```python
from build123d import *

# Parameters (mm, degrees)
BOSS_EXTRUDE1_DEPTH = 40
SKETCH2_R           = 2.1
CUT_EXTRUDE1_DEPTH  = 40
SKETCH3_R           = 2.1
CUT_EXTRUDE2_DEPTH  = 40
BOSS_EXTRUDE2_DEPTH = 4
BOSS_EXTRUDE3_DEPTH = 4


with BuildPart() as part:
    # Sketch1 → Boss-Extrude1 (new body)
    with BuildSketch(Plane(origin=(0, 0, 0), x_dir=(1, 0, 0), z_dir=(0, 1, 0))):
        Polygon((0, 0), (0, 40), (-40, 40), (-40, 36), (-4, 36), (-4, 0), align=None)
    extrude(amount=BOSS_EXTRUDE1_DEPTH)

    # Sketch2 → Cut-Extrude1 (cut)
    with BuildSketch(Plane(origin=(0, 0, -40), x_dir=(-1, 0, 0), z_dir=(0, 0, -1))):
        with Locations((30, 30)):
            Circle(SKETCH2_R)
        with Locations((30, 10)):
            Circle(SKETCH2_R)
        with Locations((10, 10)):
            Circle(SKETCH2_R)
        with Locations((10, 30)):
            Circle(SKETCH2_R)
    extrude(amount=-CUT_EXTRUDE1_DEPTH, mode=Mode.SUBTRACT)

    # Sketch3 → Cut-Extrude2 (cut)
    with BuildSketch(Plane(origin=(0, 0, 0), x_dir=(0, 0, -1), z_dir=(1, 0, 0))):
        with Locations((10, 30)):
            Circle(SKETCH3_R)
        with Locations((30, 30)):
            Circle(SKETCH3_R)
        with Locations((30, 10)):
            Circle(SKETCH3_R)
        with Locations((10, 10)):
            Circle(SKETCH3_R)
    extrude(amount=-CUT_EXTRUDE2_DEPTH, mode=Mode.SUBTRACT)

    # Sketch4 → Boss-Extrude2 (add)
    with BuildSketch(Plane(origin=(0, 40, 0), x_dir=(1, 0, 0), z_dir=(0, 1, 0))):
        Polygon((-40, 36), (-4, 0), (-4, 36), align=None)
    extrude(amount=-BOSS_EXTRUDE2_DEPTH)

    # Sketch5 → Boss-Extrude3 (add)
    with BuildSketch(Plane.XZ):
        Polygon((-4, -36), (-4, 0), (-40, -36), align=None)
    extrude(amount=-BOSS_EXTRUDE3_DEPTH)


solid = part.part
```
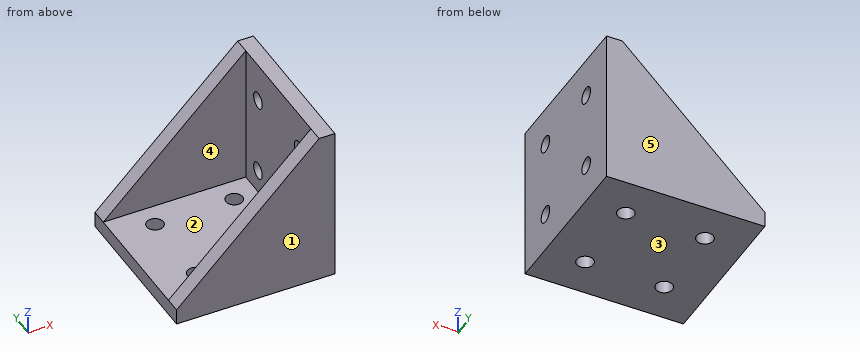
Check sheet for the modelled part. Datum: model origin and axes. Units: mm. Face numbers are marked on the shaded views. A direction names the side the tool comes from. Round coordinates to 2 decimals unless told otherwise and drop trailing zeros. Loops run counter-clockwise (first coordinate to the right, second up) from the corner with the lowest first, then second, coordinate; pieces in that order, holes last. Notation, with made-up numbers: (7.5, 14.5) -> (36.5, 14.5) arc R26 cw to (36.5, 46.5) -> close; hole circle Ø4 at (-19.5, 2.25). An arc over 180 degrees is marked (long way). Write item = value, one per line. Start each with the question number.
1) Release check for a two-part mould opening along Y. For the marked faces 3, 4 and 5 record: released by +Y, released by -Y, zero draft, split by the parting line, or undercut.
2) Thickness scan on probe 1 along Y at (x, z) = (-2.7, -30); probe 2 along Y at (x, z) = (-12, -22.5); probe 3 along X at (y, z) = (16.5, -10). Record the ranges inside material, lowest first.
3) Sectioned sample at C-C, the plane x = -30. Record the cut outline in (y, z), plus the area to 3 significant figures.
4) Set-up check for the marked faces 1 and 2: record each of +Z, -Z, +X, -X, +Y, -Y from which the full face is reachable in a straight line by a thin tool's end or side.
5) Sectioned sample at D-D, the plane x = -25. Record the cut outline in (y, z), plus the area to 3 significant figures.
6) Sectioned sample at A-A, the plane y = 10. Record the cut outline in (x, z).
7) Sectioned sample at B-B, the plane z = -10. Record the cut outline in (x, y).
8) Gauge pin test, flat ends, axial feed: pin 1 Ø10 at (x, y) = (-30, 28.5) entering from +Z; pin 2 Ø4 at (y, z) = (11, -19.5) entering from -X. Record the tip position at first contact, or that the pin passes through.
Results are:
q1.face_3 = zero draft
q1.face_4 = undercut
q1.face_5 = released by +Y
q2.probe_1 = 0 to 7.9, 12.1 to 27.9, 32.1 to 40
q2.probe_2 = 0 to 4, 36 to 40
q2.probe_3 = -4 to 0
q3.outline = (0, -40) -> (7.9, -40) -> (7.9, -36) -> (4, -36) -> (4, -26) -> (0, -26) -> close; (12.1, -40) -> (27.9, -40) -> (27.9, -36) -> (12.1, -36) -> close; (32.1, -40) -> (40, -40) -> (40, -26) -> (36, -26) -> (36, -36) -> (32.1, -36) -> close
q3.area = 206 mm^2
q4.face_1 = +Z, -Z, +X, -X, -Y
q4.face_2 = +Z, -X
q5.outline = (0, -40) -> (40, -40) -> (40, -21) -> (36, -21) -> (36, -36) -> (4, -36) -> (4, -21) -> (0, -21) -> close
q5.area = 280 mm^2
q6.outline = (-40, -40) -> (-32.1, -40) -> (-32.1, -36) -> (-40, -36) -> close; (-27.9, -40) -> (-12.1, -40) -> (-12.1, -36) -> (-27.9, -36) -> close; (-7.9, -40) -> (0, -40) -> (0, -32.1) -> (-4, -32.1) -> (-4, -36) -> (-7.9, -36) -> close; (-4, -27.9) -> (0, -27.9) -> (0, -12.1) -> (-4, -12.1) -> close; (-4, -7.9) -> (0, -7.9) -> (0, 0) -> (-4, 0) -> close
q7.outline = (-14, 0) -> (0, 0) -> (0, 7.9) -> (-4, 7.9) -> (-4, 4) -> (-14, 4) -> close; (-14, 36) -> (-4, 36) -> (-4, 32.1) -> (0, 32.1) -> (0, 40) -> (-14, 40) -> close; (-4, 12.1) -> (0, 12.1) -> (0, 27.9) -> (-4, 27.9) -> close
q8.pin_1 = -36
q8.pin_2 = -4
